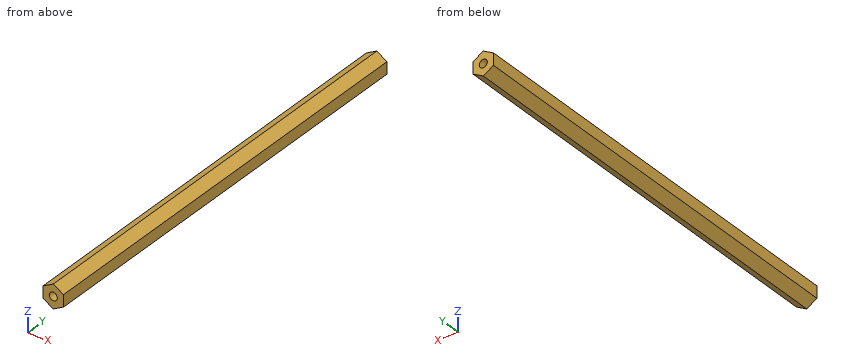
from build123d import *

# Parameters (mm, degrees)
BOSS_EXTRUDE1_DEPTH       = 130
M6X1_0_TAPPED_HOLE1_D     = 5
M6X1_0_TAPPED_HOLE1_DEPTH = 15
M6X1_0_TAPPED_HOLE1_TIP   = 1.502151548
M6X1_0_TAPPED_HOLE2_D     = 5
M6X1_0_TAPPED_HOLE2_DEPTH = 15
M6X1_0_TAPPED_HOLE2_TIP   = 1.502151548


with BuildPart() as part:
    # Sketch1 → Boss-Extrude1 (new, symmetric)
    with BuildSketch(Plane(origin=(0, 0, 0), x_dir=(1, 0, 0), z_dir=(0, 1, 0))):
        Polygon((6.349472256, -3.667088137), (6.350527612, 3.665260206), (0.001055356, 7.332348343), (-6.349472256, 3.667088137), (-6.350527612, -3.665260206), (-0.001055356, -7.332348343), align=None)
    extrude(amount=BOSS_EXTRUDE1_DEPTH, both=True)

    # M6x1.0 Tapped Hole1
    with Locations(Plane(origin=(0, 130, 0), x_dir=(1, 0, 0), z_dir=(0, 1, 0))):
        with Locations((0, 0)):
            Hole(M6X1_0_TAPPED_HOLE1_D / 2, depth=M6X1_0_TAPPED_HOLE1_DEPTH)
            with Locations((0, 0, -(M6X1_0_TAPPED_HOLE1_DEPTH + M6X1_0_TAPPED_HOLE1_TIP / 2))):  # 118° drill point
                Cone(0, M6X1_0_TAPPED_HOLE1_D / 2, M6X1_0_TAPPED_HOLE1_TIP, mode=Mode.SUBTRACT)

    # M6x1.0 Tapped Hole2
    with Locations(Plane(origin=(0, -130, 0), x_dir=(-1, 0, 0), z_dir=(0, -1, 0))):
        with Locations((0, 0)):
            Hole(M6X1_0_TAPPED_HOLE2_D / 2, depth=M6X1_0_TAPPED_HOLE2_DEPTH)
            with Locations((0, 0, -(M6X1_0_TAPPED_HOLE2_DEPTH + M6X1_0_TAPPED_HOLE2_TIP / 2))):  # 118° drill point
                Cone(0, M6X1_0_TAPPED_HOLE2_D / 2, M6X1_0_TAPPED_HOLE2_TIP, mode=Mode.SUBTRACT)


solid = part.part
Geometry: final body of the model. Coordinates: model frame, mm. Give positions to 0.01 mm unless a question says otherwise; leave off trailing zeros. Loops run counter-clockwise (first coordinate to the right, second up) from the corner with the lowest first, then second, coordinate; pieces in that order, holes last. Notation, with made-up numbers: (37.5, 60.25) - (54.5, 60.25) arc R21 cw to (54.5, 86.25) - close; hole circle Ø9 at (14, 25). An arc over 180 degrees is marked (long way). Answer as CSV lines item,"result". Start each with the question number.
1. Section A-A, the plane y = 64. Return loops of the section in (x, z).
2. Ray query, L1, parallel to Z at x = 0, y = 118.75; L2, parallel to X at y = -118, z = 0.5; L3, parallel to Z at x = -1.75, y = -92. Return the intervals inside material, ascending.
3. Pin query (flat end, axial travel): P1, Ø1, axis at x = -1.5, y = -14.5, coming from the -Z side; P2, Ø3, axis at x = 0.5, y = 81.5, coming from the -Z side; P3, Ø4, axis at x = -3.5, y = -77.5, coming from the -Z side; P4, Ø4, axis at x = 0, z = 0, coming from the -Y side. Return the tip coordinate at first contact, or that it passes through.
Answers:
1,outline,"(-6.35, -3.67) - (0, -7.33) - (6.35, -3.67) - (6.35, 3.67) - (0, 7.33) - (-6.35, 3.67) - close"
2,L1,"z = -7.33 to -2.5, 2.5 to 7.33"
2,L2,"x = -6.35 to -2.45, 2.45 to 6.35"
2,L3,"z = -6.32 to 6.32"
3,P1,"stops at z = -6.75"
3,P2,"stops at z = -7.33"
3,P3,"stops at z = -6.47"
3,P4,"stops at y = -114.7"
